Autodesk Fusion 360 part; units mm, degrees
sketch "スケッチ1" plane through (0, 0, 0) normal (0, 0, 1) x (1, 0, 0)
  line L0 (-3.5, 163) -> (-86.5, 163)
  line L1 (-86.5, 163) -> (-86.5, -163)
  line L2 (-86.5, -163) -> (-3.5, -163)
  line L3 (86.5, -125) -> (86.5, 155)
  line L4 (82.2546, 155) -> (-86.5, -163) construction
  line L5 (-86.5, 163) -> (70.0256, -131.9558) construction
  line L6 (-3.5, 163) -> (-3.5, 155)
  line L7 (-3.5, 155) -> (86.5, 155)
  line L8 (-86.5, -163) -> (-3.5, -163) construction
  line L9 (-3.5, -163) -> (86.5, -125)
  dimension "d2" = 326
  dimension "d5" = 83
extrude "押し出し1" add sketch "スケッチ1" along normal blind 8
chamfer "面取り1" distance 30 angle 45 2 edges at (-86.5, -163, 4) (-86.5, 163, 4)
sketch "スケッチ2" plane through (0, 0, 8) normal (0, 0, 1) x (-1, 0, 0)
  line L0 (56.5, -163) -> (86.5, -133)
  line L1 (86.5, -133) -> (86.5, 133)
  line L2 (86.5, 133) -> (56.5, 163)
  line L3 (56.5, 163) -> (3.5, 163)
  line L4 (3.5, 163) -> (-86.5, 125)
  line L5 (-86.5, 125) -> (-86.5, -155)
  line L6 (-86.5, -155) -> (3.5, -155)
  line L7 (3.5, -155) -> (3.5, -163)
  line L8 (3.5, -163) -> (56.5, -163)
  line L9 (-86.5, -155) -> (-46.5, -155) construction
  line L10 (-46.5, -155) -> (-46.5, -95) construction
  line L11 (-46.5, -95) -> (-86.5, -95) construction
  line L12 (-86.5, -95) -> (-86.5, -155) construction
  line L13 (-46.5, -95) -> (-46.5, -25) construction
  line L14 (-46.5, -25) -> (-46.5, 45) construction
  point P0 (-46.5, -95)
  point P1 (-46.5, -25)
  point P2 (-46.5, 45)
  dimension "d10" = 40
  dimension "d11" = 60
  dimension "d12" = 70
  dimension "d13" = 70
hole "穴1" at (46.5, 95, 8) at (46.5, 25, 8) at (46.5, -45, 8) direction (0, 0, -1) diameter 22 end through all
equation "d5 = 30 mm + 53 mm"
Build history of the part. All positions in model axes, mm. A direction names the side the tool comes from. Give positions to 0.01 mm unless a question says otherwise; leave off trailing zeros. Loops run counter-clockwise (first coordinate to the right, second up) from the corner with the lowest first, then second, coordinate; pieces in that order, holes last. Notation, with made-up numbers: (88, -11.5) -> (103, -11.5) arc R26 ccw to (103, 6.5) -> close; hole circle Ø11 at (15, 85.5). An arc over 180 degrees is marked (long way). Answer in a Markdown table with one row per item.
Item 1: Slice it at A-A on y = 25. Write the cut outline in (x, z).
Findings below:
| item | result |
|---|---|
| outline | (-86.5, 0) -> (35.5, 0) -> (35.5, 8) -> (-86.5, 8) -> close; (57.5, 0) -> (86.5, 0) -> (86.5, 8) -> (57.5, 8) -> close |
Item 2: Slice it at C-C on x = 46.5. Write the cut outline in (y, z).
Findings below:
| item | result |
|---|---|
| outline | (-141.89, 0) -> (-56, 0) -> (-56, 8) -> (-141.89, 8) -> close; (-34, 0) -> (14, 0) -> (14, 8) -> (-34, 8) -> close; (36, 0) -> (84, 0) -> (84, 8) -> (36, 8) -> close; (106, 0) -> (155, 0) -> (155, 8) -> (106, 8) -> close |
Item 3: Mould opens along X. For faces 1 (the flat face through (-3.5, 159, 4)), 2 (the cylindrical face through (46.02, 105.99, 3.94)), 3 (the flat face through (-1, 2, 0)) say: pulls with the +X half, pulls with the -X half, needs draft (parallel to the pull), parting line crosses it, or undercut.
Findings below:
| item | result |
|---|---|
| face 1 | pulls with the +X half |
| face 2 | undercut |
| face 3 | needs draft |
Item 4: Slice it at D-D on x = -62.5. Write the cut outline in (y, z), plus the area to 3 significant figures.
Findings below:
| item | result |
|---|---|
| outline | (-157, 0) -> (157, 0) -> (157, 8) -> (-157, 8) -> close |
| area | 2,510 mm² |
Item 5: Probe line 1 along X through (y, z) = (25, 3); line 2 along Y through (x, z) = (45.5, 2.5); line 3 along Y through (x, z) = (46.5, 4). List the from-to ranges inside material, lowest first. Write a range as [from, to].
Findings below:
| item | result |
|---|---|
| line 1 | x = [-86.5, 35.5], [57.5, 86.5] |
| line 2 | y = [-142.31, -55.95], [-34.05, 14.05], [35.95, 84.05], [105.95, 155] |
| line 3 | y = [-141.89, -56], [-34, 14], [36, 84], [106, 155] |
Item 6: Flat gauge pins, fed straight in: P1, Ø4, axis at x = 23.5, z = 1.5, coming from the +Y side; P2, Ø2.5, axis at y = 157.5, z = 6, coming from the +X side. Where does each tip first touch, or does it go through?
Findings below:
| item | result |
|---|---|
| P1 | stops at y = 155 |
| P2 | stops at x = -3.5 |
Item 7: Slice it at B-B on z = 6.25. Write the cut outline in (x, y), plus the area to 3 significant figures.
Findings below:
| item | result |
|---|---|
| outline | (-86.5, -133) -> (-56.5, -163) -> (-3.5, -163) -> (86.5, -125) -> (86.5, 155) -> (-3.5, 155) -> (-3.5, 163) -> (-56.5, 163) -> (-86.5, 133) -> close; hole circle Ø22 at (46.5, -45); hole circle Ø22 at (46.5, 25); hole circle Ø22 at (46.5, 95) |
| area | 51,900 mm² |
Item 8: Tool access for faces 4 (the flat face through (40.87, -144.266, 3.944)), 5 (the flat face through (41, 155, 4)): list every direction of +Z, -Z, +X, -X, +Y, -Y with a clear straight run to the whole face (end or side of a thin tool).
Findings below:
| item | result |
|---|---|
| face 4 | +Z, -Z, +X, -Y |
| face 5 | +Z, -Z, +X, +Y |
